Build history of the part. All positions in model axes, mm. A direction names the side the tool comes from. Give positions to 0.01 mm unless a question says otherwise; leave off trailing zeros. Order: outer loops, then holes, each group sorted by start corner. A loop starts at its lowest first (then second) coordinate and runs counter-clockwise, first axis right, second up. Notation, with made-up numbers: M 85,10 L 108,10 A11 ccw 108,19 Z; hole C 41,-31 d2. An arc over 180 degrees is marked long. Answer as CSV lines item,"result".
from build123d import *

# Parameters (mm, degrees)
SKETCH1_W           = 50
SKETCH1_H           = 15.1
BOSS_EXTRUDE1_DEPTH = 2.5
SKETCH3_R           = 1.5
CUT_EXTRUDE1_DEPTH  = 3.5
SKETCH4_W           = 2.5
SKETCH4_H           = 15.1
BOSS_EXTRUDE2_DEPTH = 50
SKETCH6_R           = 1
CUT_EXTRUDE2_DEPTH  = 45
SKETCH8_W           = 47.5
SKETCH8_H           = 2
BOSS_EXTRUDE3_DEPTH = 50
CUT_EXTRUDE3_DEPTH  = 3


with BuildPart() as part:
    # Sketch1 → Boss-Extrude1 (new body)
    with BuildSketch(Plane(origin=(0, 0, 0), x_dir=(0, 0, -1), z_dir=(1, 0, 0))):
        with Locations((25, 7.55)):
            Rectangle(SKETCH1_W, SKETCH1_H)
    extrude(amount=BOSS_EXTRUDE1_DEPTH)

    # Sketch3 → Cut-Extrude1 (cut, through all)
    with BuildSketch(Plane(origin=(2.5, 0, 0), x_dir=(0, 0, -1), z_dir=(1, 0, 0))):
        with Locations((46, 8.55)):
            Circle(SKETCH3_R)
        with Locations((9, 8.55)):
            Circle(SKETCH3_R)
    extrude(amount=-CUT_EXTRUDE1_DEPTH, mode=Mode.SUBTRACT)

    # Sketch4 → Boss-Extrude2 (add)
    with BuildSketch(Plane(origin=(2.5, 0, 0), x_dir=(0, 0, -1), z_dir=(1, 0, 0))):
        with Locations((1.25, 7.55)):
            Rectangle(SKETCH4_W, SKETCH4_H)
    extrude(amount=BOSS_EXTRUDE2_DEPTH)

    # Sketch6 → Cut-Extrude2 (cut)
    with BuildSketch(Plane(origin=(0, 0, -2.5), x_dir=(-1, 0, 0), z_dir=(0, 0, -1))):
        with Locations((-7.5, 8.55)):
            Circle(SKETCH6_R)
        with Locations((-10.6, 8.55)):
            Circle(SKETCH6_R)
        with Locations((-13.7, 8.55)):
            Circle(SKETCH6_R)
        with Locations((-16.8, 8.55)):
            Circle(SKETCH6_R)
        with Locations((-19.9, 8.55)):
            Circle(SKETCH6_R)
        with Locations((-35.2, 8.55)):
            Circle(SKETCH6_R)
        with Locations((-38.3, 8.55)):
            Circle(SKETCH6_R)
        with Locations((-41.4, 8.55)):
            Circle(SKETCH6_R)
        with Locations((-44.5, 8.55)):
            Circle(SKETCH6_R)
        with Locations((-47.6, 8.55)):
            Circle(SKETCH6_R)
    extrude(amount=-CUT_EXTRUDE2_DEPTH, mode=Mode.SUBTRACT)

    # Sketch8 → Boss-Extrude3 (add)
    with BuildSketch(Plane(origin=(2.5, 0, 0), x_dir=(0, 0, -1), z_dir=(1, 0, 0))):
        with Locations((26.25, 1)):
            Rectangle(SKETCH8_W, SKETCH8_H)
    extrude(amount=BOSS_EXTRUDE3_DEPTH)

    # Sketch9 → Cut-Extrude3 (cut, through all)
    with BuildSketch(Plane(origin=(0, 2, 0), x_dir=(1, 0, 0), z_dir=(0, 1, 0))):
        Polygon((45.240466198, 2.5), (2.5, 43.103442888), (2.5, 23.646557112), (24.759533802, 2.5), align=None)
        Polygon((52.5, 2.5), (2.5, 50), (52.5, 50), align=None)
        Polygon((17.5, 2.5), (2.5, 16.75), (2.5, 2.5), align=None)
    extrude(amount=-CUT_EXTRUDE3_DEPTH, mode=Mode.SUBTRACT)


solid = part.part
Item 1: Band-saw the part on A-A (x = 16.8). Give the cut face in (y, z) (3 decimals), and give its area (3 significant figures).
Geometry says:
outline,"M 0,-36.415 L 2,-36.415 L 2,-29.518 L 0,-29.518 Z; M 0,-10.062 L 2,-10.062 L 2,-3.165 L 0,-3.165 Z; M 0,-2.5 L 7.55,-2.5 L 7.55,0 L 0,0 Z; M 9.55,-2.5 L 15.1,-2.5 L 15.1,0 L 9.55,0 Z"
area,"60.3 mm2"
Item 2: Probe line 1 along X through (y, z) = (1, -11); line 2 along Z through (x, y) = (36, 9.5); line 3 along Y through (x, z) = (38.3, -0.75). List the from-to ranges inside material, lowest first. Write a range as from..to.
Geometry says:
line 1,"x = 0..2.5, 8.55..15.81, 36.29..43.55"
line 2,"z = -2.5..0"
line 3,"y = 0..7.55, 9.55..15.1"
Item 3: Band-saw the part on B-B (z = -6). Give the cut face in (x, y).
Geometry says:
outline,"M 0,0 L 2.5,0 L 2.5,15.1 L 0,15.1 Z; M 13.82,0 L 21.08,0 L 21.08,2 L 13.82,2 Z; M 41.56,0 L 48.82,0 L 48.82,2 L 41.56,2 Z"
Item 4: Drop flat-ended pins along their axis: pin 1 (1.8 mm diameter, centred on x = 41.4, y = 8.55, fed in from +Z); pin 2 (3 mm diameter, centred on x = 7.5, y = 8.55, fed in from -Z); pin 3 (5 mm diameter, centred on y = 11, z = -16, fed in from +X); pin 4 (10.5 mm diameter, centred on x = 15, z = -10.5, fed in from +Y). Give the stop position or say it passes through.
Geometry says:
pin 1,"passes through"
pin 2,"stops at z = -2.5"
pin 3,"stops at x = 2.5"
pin 4,"stops at y = 2"
Item 5: 3-axis set-ups, long thin cutter, end or side, ignore diameter. For faces 4 (the flat face through (14, 15.1, -1)), 5 (the flat face through (12, 2, -12)), 6 (the flat face through (13.474, 1.014, -13.221)): which of +Z, -Z, +X, -X, +Y, -Y reach the whole face in a straight line?
Geometry says:
face 4,"+Z, -Z, +X, -X, +Y"
face 5,"-Z, +X, +Y"
face 6,"+Y, -Y"
Item 6: Pull direction Y, two halves, no side cores. Call faces 1 (the flat face through (1, 7, -50)), 2 (the flat face through (27, 2, -24)), 3 (the cylindrical face through (12.776, 8.167, -1.268)): released by +Y, released by -Y, zero draft, split by the parting line, or undercut.
Geometry says:
face 1,"zero draft"
face 2,"released by +Y"
face 3,"undercut"
Item 7: Band-saw the part on C-C (x = 32.5). Give the cut face in (y, z), and give its area (3 significant figures).
Geometry says:
outline,"M 0,-21.5 L 2,-21.5 L 2,-14.6 L 0,-14.6 Z; M 0,-2.5 L 15.1,-2.5 L 15.1,0 L 0,0 Z"
area,"51.5 mm2"
Item 8: Band-saw the part on D-D (z = -22). Give the cut face in (x, y), and give its area (3 significant figures).
Geometry says:
outline,"M 0,0 L 4.23,0 L 4.23,2 L 2.5,2 L 2.5,15.1 L 0,15.1 Z; M 24.71,0 L 31.97,0 L 31.97,2 L 24.71,2 Z"
area,"55.7 mm2"
